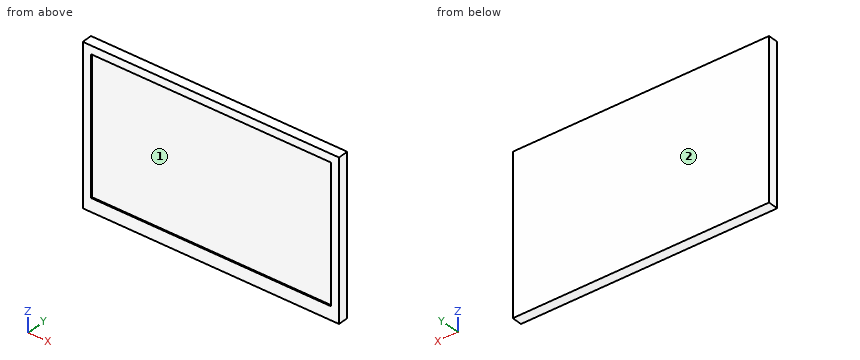
```python
from build123d import *

# Parameters (mm, degrees)
SKETCH_W     = 1000
SKETCH_H     = 615
PAD_DEPTH    = 40
SKETCH001_W  = 936
SKETCH001_H  = 531
POCKET_DEPTH = 5


with BuildPart() as part:
    # Sketch → Pad (new body)
    with BuildSketch(Plane.XZ):
        Rectangle(SKETCH_W, SKETCH_H)
    extrude(amount=PAD_DEPTH)

    # Sketch001 (on Face6 of Pad) → Pocket (cut)
    with BuildSketch(Plane.XZ.offset(40)):
        with Locations((0, 10)):
            Rectangle(SKETCH001_W, SKETCH001_H)
    extrude(amount=-POCKET_DEPTH, mode=Mode.SUBTRACT)


solid = part.part
```
The model under review builds one solid part; all positions refer to its coordinate system, in mm. Face numbers are marked on the shaded views. Coordinates: 2 decimals unless noted, no trailing zeros. Write each loop counter-clockwise with the first axis right and the second up, starting at its lowest first coordinate (ties: lowest second). Pieces come first, ordered by that corner, then holes.
1) Clearance check with flat-ended pins moving along their axes: pin 1 Ø1.5 at (x, z) = (-12.5, 68.5) entering from +Y; pin 2 Ø2 at (x, z) = (-125.5, 127) entering from -Y. State where each tip first meets the part, or that it passes through.
2) To check wall thickness, follow probe 1 along Z at (x, y) = (317, -37); probe 2 along Y at (x, z) = (-367, -49). State the ranges of each line that lie inside material, in increasing order.
3) We need section B-B on x = -389. State the section outline as (y, z) points.
4) We need section A-A on z = 10. State the section outline as (x, y) points.
5) The part is to be moulded in two halves that separate along X. For the marked faces 1 and 2, say which applies: pulls with the +X half, pulls with the -X half, needs draft (parallel to the pull), parting line crosses it, or undercut.
Answer list:
1. pin 1: stops at y = 0
1. pin 2: stops at y = -35
2. probe 1: z = -307.5 to -255.5, 275.5 to 307.5
2. probe 2: y = -35 to 0
3. outline: (-40, -307.5) - (0, -307.5) - (0, 307.5) - (-40, 307.5) - (-40, 275.5) - (-35, 275.5) - (-35, -255.5) - (-40, -255.5) - close
4. outline: (-500, -40) - (-468, -40) - (-468, -35) - (468, -35) - (468, -40) - (500, -40) - (500, 0) - (-500, 0) - close
5. face 1: undercut
5. face 2: needs draft
